```python
from build123d import *

# Parameters (mm, degrees)
F0_W     = 38.1
F0_H     = 50.8
F1_DEPTH = 25.4
F2_R     = 5.321042
F3_DEPTH = 25.4
F4_R     = 5.08


with BuildPart() as f1:
    # F0 (on Top) → F1 (new body)
    with BuildSketch(Plane.XY):
        Rectangle(F0_W, F0_H)
    extrude(amount=F1_DEPTH)

    # F2 (on face) → F3 (join)
    with BuildSketch(Plane.XY.offset(25.4)):
        with Locations((-9.905285, 6.918165)):
            Circle(F2_R)
    extrude(amount=F3_DEPTH)

    # F4
    f4_edges = [f1.edges().sort_by_distance(p)[0] for p in [
        (-19.05, -25.4, 12.7),
        (19.05, -25.4, 12.7),
        (-19.05, 25.4, 12.7),
        (19.05, 25.4, 12.7),
    ]]
    fillet(f4_edges, radius=F4_R)


solid = f1.part
```
The listing builds one solid part. Answer for the finished solid, in the listing's coordinates (mm). A direction names the side the tool comes from. Round coordinates to 2 decimals unless told otherwise and drop trailing zeros. Loops run counter-clockwise (first coordinate to the right, second up) from the corner with the lowest first, then second, coordinate; pieces in that order, holes last.
Q1. Section D-D, the plane y = -19.5 is taken. Determine the outline of the cut face in (x, z).
Q2. Section A-A, the plane x = -7.5 is taken. Determine the outline of the cut face in (y, z), then the cut area to 3 significant figures.
Q3. Section C-C, the plane z = 45 is taken. Determine the outline of the cut face in (x, y), then the cut area to 3 significant figures.
Q4. Section B-B, the plane y = 3.5 is taken. Determine the outline of the cut face in (x, z).
Q5. Given pin 1 Ø12 at (x, z) = (1, 35) entering from +Y; pin 2 Ø19 at (x, y) = (1.5, -7) entering from +Z, each flat-ended and moving along its own axis, determine where each tip first touches the part or whether it passes through.
Q6. Which of the six approach directions +Z, -Z, +X, -X, +Y, -Y give full straight-line access (tool end or side, diameter ignored) to faces 1 (the face through (-10.598, 12.194, 37.922)), 2 (the face through (-19.05, 0, 13))?
Q7. Find the intervals of material crossed by line 1 (Z direction, x = 0, y = 2.5); line 2 (X direction, y = 2, z = 27); line 3 (Y direction, x = 16.5, z = 12.5), in increasing order.
Completed:
1. outline: (-19.05, 0) - (19.05, 0) - (19.05, 25.4) - (-19.05, 25.4) - close
2. outline: (-25.4, 0) - (25.4, 0) - (25.4, 25.4) - (11.66, 25.4) - (11.66, 50.8) - (2.17, 50.8) - (2.17, 25.4) - (-25.4, 25.4) - close
2. area: 1,530 mm2
3. outline: circle Ø10.64 at (-9.91, 6.92)
3. area: 88.9 mm2
4. outline: (-19.05, 0) - (19.05, 0) - (19.05, 25.4) - (-5.83, 25.4) - (-5.83, 50.8) - (-13.98, 50.8) - (-13.98, 25.4) - (-19.05, 25.4) - close
5. pin 1: stops at y = 8.98
5. pin 2: stops at z = 25.4
6. face 1: +Z
6. face 2: +Z, -Z, -X, +Y, -Y
7. line 1: z = 0 to 25.4
7. line 2: x = -11.94 to -7.87
7. line 3: y = -24.73 to 24.73
